Drawing for the job (mm, zero at the part's lowest x, y, z). Coordinates: 2 decimals unless noted, no trailing zeros. Write each loop counter-clockwise with the first axis right and the second up, starting at its lowest first coordinate (ties: lowest second). Pieces come first, ordered by that corner, then holes.
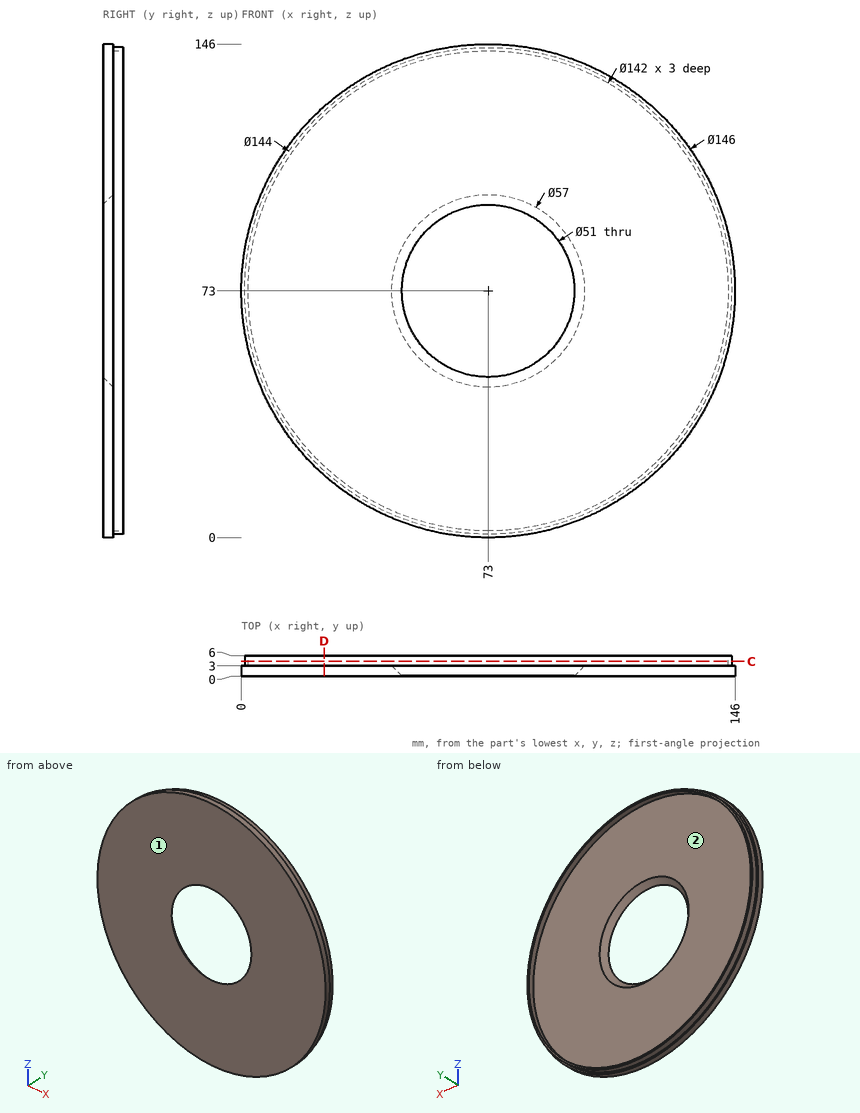
Item 1: Wall check: line 1 along X through (y, z) = (3.6, 73); line 2 along Y through (x, z) = (18, 43.5); line 3 along X through (y, z) = (5.55, 66). Give the ranges that are in metal, low to high.
Item 2: Two-plate mould, pull along X, no slides. Class the marked faces 1 and 2: +X half, -X half, draft (parallel to the pull), parting line (faces both ways), or undercut.
Item 3: Saw through at D-D, the plane x = 24.5. Write the cut outline in (y, z).
Item 4: Saw through at C-C, the plane y = 4.35. Write the cut outline in (x, z).
Item 5: Flat gauge pins, fed straight in: pin 1 Ø1 at (x, z) = (86.5, 41.5) entering from -Y; pin 2 Ø1.5 at (y, z) = (5, 113.5) entering from +X; pin 3 Ø3 at (x, y) = (95.5, 3.5) entering from +Z; pin 4 Ø1.5 at (y, z) = (2.5, 83.5) entering from -X. Where does each tip first touch, or does it go through?
Working result:
1. line 1: x = 1 to 2, 144 to 145
1. line 2: y = 0 to 3
1. line 3: x = 1.34 to 2.35, 143.65 to 144.66
2. face 1: draft
2. face 2: undercut
3. outline: (0, 18.44) - (3, 18.44) - (3, 19.79) - (6, 19.79) - (6, 21.15) - (3, 21.15) - (3, 124.85) - (6, 124.85) - (6, 126.21) - (3, 126.21) - (3, 127.56) - (0, 127.56) - close
4. outline: circle Ø144 at (73, 73); hole circle Ø142 at (73, 73)
5. pin 1: stops at y = 0
5. pin 2: stops at x = 133.03
5. pin 3: stops at z = 142.89
5. pin 4: stops at x = 0.65
